Model file for the job. Use its own axes, mm. A direction names the side the tool comes from. Coordinates: 2 decimals unless noted, no trailing zeros. Write each loop counter-clockwise with the first axis right and the second up, starting at its lowest first coordinate (ties: lowest second). Pieces come first, ordered by that corner, then holes. Notation, with made-up numbers: (38.5, 81) - (57.5, 81) arc R25 ccw to (57.5, 98) - close; hole circle Ø5 at (72.25, -20.5). An arc over 180 degrees is marked (long way). Put each result on its own line as item: value. Start each with the question number.
1. Which spindle directions (+Z, -Z, +X, -X, +Y, -Y) get a long thin tool onto all of the face, cutting with end or side? Do faces 1 (the face through (-0.1, 9.8, -0.3)), 2 (the face through (3.905, 14.305, 0.867)). Say none if no direction does.
2. Saw through at D-D, the plane y = 14.5. Write the cut outline in (x, z), plus the area to 3 significant figures.
3. Drop flat-ended pins along their axis: P1, Ø4, axis at x = 2.5, z = 3.5, coming from the +Y side; P2, Ø3, axis at x = -2.5, y = 13.5, coming from the +Z side; P3, Ø1, axis at x = -2.5, y = 10, coming from the -Z side; P4, Ø3, axis at x = 0, z = 0, coming from the -Y side. Give the stop position or say it passes through.
4. Pull direction X, two halves, no side cores. Call faces 3 (the face through (1.216, 4.563, 1.115)), 4 (the face through (-5.5, 3, 0)), 5 (the face through (-1.3, 0, -1.3)): released by +X, released by -X, zero draft, split by the parting line, or undercut.
5. Drill centre lines: L1, parallel to Z at x = 0, y = 3; L2, parallel to X at y = 8, z = 0. Where is each one in solid material? Low to high. Write a range as from..to.
6. Saw through at B-B, the plane x = -3.75. Write the cut outline in (y, z), plus the area to 3 significant figures.
7. Saw through at C-C, the plane z = 2.75. Write the cut outline in (x, y).
8. Saw through at A-A, the plane y = 7.25. Write the cut outline in (x, z), plus the area to 3 significant figures.
```python
from build123d import *

# Parameters (mm, degrees)
ESQUISSE2_OUTSIDE_W     = 24.27
ESQUISSE2_OUTSIDE_H     = 24.27
ESQUISSE2_OUTSIDE_W_2   = 11
ESQUISSE2_OUTSIDE_H_2   = 11
ENL_V_MAT_EXTRU_1_DEPTH = 25.472229159
TROU_TARAUD_M41_D       = 3.3
TROU_TARAUD_M41_DEPTH   = 9
TROU_TARAUD_M41_TIP     = 0.991420021


with BuildPart() as part:
    # Esquisse1 → Révolution1 (revolve)
    with BuildSketch(Plane.XY, mode=Mode.PRIVATE) as r_volution1_sk:
        Polygon((0, 0), (8, 0), (8, 6.7), (4, 6.7), (4, 21.7), (0, 21.7), align=None)
    revolve(r_volution1_sk.sketch.rotate(Axis((0, 0, 0), (0, 1, 0)), 90), axis=Axis((0, 0, 0), (0, 1, 0)))

    # Esquisse2 outside → Enlèv. mat.-Extru.1 (cut, through all)
    with BuildSketch(Plane.XZ):
        Rectangle(ESQUISSE2_OUTSIDE_W, ESQUISSE2_OUTSIDE_H)
        Rectangle(ESQUISSE2_OUTSIDE_W_2, ESQUISSE2_OUTSIDE_H_2, mode=Mode.SUBTRACT)
    extrude(amount=-ENL_V_MAT_EXTRU_1_DEPTH, mode=Mode.SUBTRACT)

    # Trou taraudé M41
    with Locations(Plane.XZ):
        with Locations((0, 0)):
            Hole(TROU_TARAUD_M41_D / 2, depth=TROU_TARAUD_M41_DEPTH)
            with Locations((0, 0, -(TROU_TARAUD_M41_DEPTH + TROU_TARAUD_M41_TIP / 2))):  # 118° drill point
                Cone(0, TROU_TARAUD_M41_D / 2, TROU_TARAUD_M41_TIP, mode=Mode.SUBTRACT)


solid = part.part
```
Final values:
1. face 1: -Y
1. face 2: +Y
2. outline: circle Ø8 at (0, 0)
2. area: 50.3 mm²
3. P1: stops at y = 21.7
3. P2: stops at z = 3.87
3. P3: stops at z = -3.46
3. P4: stops at y = 9.09
4. face 3: undercut
4. face 4: released by -X
4. face 5: zero draft
5. L1: z = -5.5..-1.65, 1.65..5.5
5. L2: x = -4..-1.65, 1.65..4
6. outline: (0, -5.5) - (6.7, -5.5) - (6.7, -1.39) - (21.7, -1.39) - (21.7, 1.39) - (6.7, 1.39) - (6.7, 5.5) - (0, 5.5) - close
6. area: 115 mm²
7. outline: (-5.5, 0) - (5.5, 0) - (5.5, 6.7) - (2.9, 6.7) - (2.9, 21.7) - (-2.9, 21.7) - (-2.9, 6.7) - (-5.5, 6.7) - close
8. outline: circle Ø8 at (0, 0); hole circle Ø3.3 at (0, 0)
8. area: 41.7 mm²
